Check sheet for the modelled part. Datum: model origin and axes. Units: mm. A direction names the side the tool comes from. Coordinates: 2 decimals unless noted, no trailing zeros. Write each loop counter-clockwise with the first axis right and the second up, starting at its lowest first coordinate (ties: lowest second). Pieces come first, ordered by that corner, then holes. Notation, with made-up numbers: (69, -3.5) - (97, -3.5) arc R14 ccw to (97, 11.5) - close; hole circle Ø9 at (43, 7). An arc over 180 degrees is marked (long way). Write each question's results on one line, items separated by ' | '.
from build123d import *

# Parameters (mm, degrees)
EXTRUDE_1_DEPTH          = 5
SKETCH_3_R               = 2
SKETCH_3_R_2             = 1
EXTRUDE_2_DEPTH          = 4
EXTRUDE_2_DEPTH_BACK     = 14
CUT_EXTRUDE_1_DEPTH      = 4
SKETCH_4_W               = 2.59101906
SKETCH_4_H               = 1.951015164
SKETCH_4_H_2             = 2.185859581
CUT_EXTRUDE_2_DEPTH      = 1
CUT_EXTRUDE_2_DEPTH_BACK = 22.850089698
SKETCH_5_W               = 31.280846128
SKETCH_5_H               = 26.509191634
CUT_EXTRUDE_3_DEPTH      = 10
CUT_EXTRUDE_4_DEPTH      = 10
EXTRUDE_4_DEPTH          = 10


with BuildPart() as part:
    # 草图1 → 凸台-拉伸1 (new body, symmetric)
    with BuildSketch(Plane.XY):
        with BuildLine():
            Line((-11, -0.656322646), (-11, -22.429975294))
            ThreePointArc((-11, -22.429975294), (-16.212842401, -27.826367541), (-21.786325372, -22.803314409))
            add(Edge.make_bspline(
                [(-20.992129713, -14.197793305), (-22.083985192, -18.508547069), (-21.786325372, -22.803314409)],
                knots=[0, 0, 0, 0.849528989, 0.849528989, 0.849528989], degree=2))
            add(Edge.make_bspline(
                [(-20.992129713, -14.197793305), (-19.982477614, -1.835246339), (-16.911295032, 22.315403308), (-5.101083491, 23.268557164)],
                knots=[0.325260196, 0.325260196, 0.325260196, 0.325260196, 1, 1, 1, 1], degree=3))
            Line((-5.101083491, 23.268557164), (-5.101083491, 16.3035208))
            ThreePointArc((-5.101083491, 16.3035208), (-5.344239377, 14.111719499), (-6.061882079, 12.026508076))
            Line((-6.061882079, 12.026508076), (-10.039201412, 3.620690077))
            ThreePointArc((-10.039201412, 3.620690077), (-10.756844114, 1.535478654), (-11, -0.656322646))
        make_face()
    extrude(amount=EXTRUDE_1_DEPTH, both=True)

    # 草图3 → 凸台-拉伸2 (add, two sides)
    with BuildSketch(Plane.XY.offset(5)) as extrude_2_sk:
        with Locations((-16.399623741, -22.429975294)):
            Circle(SKETCH_3_R)
        with Locations((-14.366531857, 0.706079338)):
            Circle(SKETCH_3_R_2)
    extrude(amount=EXTRUDE_2_DEPTH)
    extrude(extrude_2_sk.sketch, amount=-EXTRUDE_2_DEPTH_BACK)

    # 草图2 → 切除-拉伸1 (cut, symmetric)
    with BuildSketch(Plane.XY):
        with BuildLine():
            Line((-14.16063588, 12.808117781), (14.16063588, 12.808117781))
            add(Edge.make_bspline(
                [(14.16063588, 12.808117781), (18.7957473, 3.012389753), (18.151937314, -8.213759494), (19.7286529, -18.675237718)],
                knots=[0, 0, 0, 0, 1, 1, 1, 1], degree=3))
            Line((19.7286529, -18.675237718), (-19.7286529, -18.675237718))
            add(Edge.make_bspline(
                [(-14.16063588, 12.808117781), (-18.7957473, 3.012389753), (-18.151937314, -8.213759494), (-19.7286529, -18.675237718)],
                knots=[0, 0, 0, 0, 1, 1, 1, 1], degree=3))
        make_face()
    extrude(amount=CUT_EXTRUDE_1_DEPTH, both=True, mode=Mode.SUBTRACT)

    # 草图4 → 切除-拉伸2 (cut, two sides)
    with BuildSketch(Plane(origin=(0, 0, 0), x_dir=(0, 0, -1), z_dir=(1, 0, 0))) as cut_extrude_2_sk:
        with Locations((-6.29550953, -20.454467712)):
            Rectangle(SKETCH_4_W, SKETCH_4_H)
        with Locations((-6.29550953, -24.522905085)):
            Rectangle(SKETCH_4_W, SKETCH_4_H_2)
        with Locations((6.29550953, -24.522905085)):
            Rectangle(SKETCH_4_W, SKETCH_4_H_2)
        with Locations((6.29550953, -20.454467712)):
            Rectangle(SKETCH_4_W, SKETCH_4_H)
    extrude(amount=CUT_EXTRUDE_2_DEPTH, mode=Mode.SUBTRACT)
    extrude(cut_extrude_2_sk.sketch, amount=-CUT_EXTRUDE_2_DEPTH_BACK, mode=Mode.SUBTRACT)

    # 草图5 → 切除-拉伸3 (cut)
    with BuildSketch(Plane.XY.offset(5)):
        with Locations((-12.035980348, 17.707965105)):
            Rectangle(SKETCH_5_W, SKETCH_5_H)
    extrude(amount=-CUT_EXTRUDE_3_DEPTH, mode=Mode.SUBTRACT)

    # 草图6 → 切除-拉伸4 (cut)
    with BuildSketch(Plane.XY.offset(5)):
        with BuildLine():
            Line((-11, -1.030772695), (-7.289425252, 0))
            Line((-7.289425252, 0), (-6.627618858, 7.054774986))
            Line((-6.627618858, 7.054774986), (-15.000908449, 5.846258962))
            Line((-15.000908449, 5.846258962), (-16.238198664, 4.453369288))
            add(Edge.make_bspline(
                [(-16.238198664, 4.453369288), (-11.717955923, 3.797110984), (-11, -1.030772695)],
                knots=[0, 0, 0, 1, 1, 1], degree=2))
        make_face()
    extrude(amount=-CUT_EXTRUDE_4_DEPTH, mode=Mode.SUBTRACT)

    # 草图7 → 凸台-拉伸4 (add)
    with BuildSketch(Plane.XY.offset(5)):
        Polygon((-18.271249604, 4.453369288), (-18.271249604, 41.616361527), (-15.271249597, 41.616361527), (-15.271249604, 4.25345908), align=None)
    extrude(amount=-EXTRUDE_4_DEPTH)


solid = part.part
1. Access from +Z, -Z, +X, -X, +Y, -Y to the whole of each face (thin tool, end or side, straight path). Record for faces 5 (the cylindrical face through (-14.5, -21.8, -7.4)), 6 (the flat face through (-15.271, 23, 0)), 7 (the cylindrical face through (-14.5, -21.8, 7.4)), 8 (the flat face through (-11, -19, 0)), 9 (the flat face through (-16, -21.43, -6)).
Values follow:
face 5: -Z | face 6: +Z, -Z, +X, +Y | face 7: +Z | face 8: +Z, -Z, +X, +Y, -Y | face 9: +X, -X
2. Draft check along Z on faces 1 (the flat face through (-14, 1, -9)), 2 (the cylindrical face through (-15.366, 0.75, 6.972)), 3 (the flat face through (-14, 1, 9)), 4 (the flat face through (-15, -7, 4)). Enter one of: pulls with the +Z half, pulls with the -Z half, needs draft (parallel to the pull), parting line crosses it, or undercut.
Values follow:
face 1: pulls with the -Z half | face 2: needs draft | face 3: pulls with the +Z half | face 4: undercut
3. Sectioned sample at B-B (z = 6.25). Record the cut outline in (x, y), then the cut area to 3 significant figures.
Values follow:
outline: (-18.13, -23.43) - (-14.67, -23.43) arc R2 ccw to (-14.67, -21.43) - (-18.13, -21.43) arc R2 ccw to start; circle Ø2 at (-14.37, 0.71) | area: 10.8 mm^2
4. Material ranges on L1, parallel to Z at x = -12, y = -10; L2, parallel to Z at x = -16.25, y = 10; L3, parallel to Y at x = -16.25, z = -3, recorded low to high. Write a range as [from, to].
Values follow:
L1: z = [-5, -4], [4, 5] | L2: z = [-5, 5] | L3: y = [-27.83, -18.68], [4.32, 41.62]
5. Go/stop test with flat-tipped pins: pin 1 (4 mm diameter, centred on x = -15, z = 0.5, fed in from +Y); pin 2 (2.5 mm diameter, centred on x = -14.5, y = -9, fed in from -Z); pin 3 (3 mm diameter, centred on y = 32, z = -2, fed in from -X); pin 4 (5 mm diameter, centred on x = -19.5, z = -4, fed in from -Y). Record where each tip stops, or that it passes through.
Values follow:
pin 1: stops at y = 41.62 | pin 2: stops at z = -5 | pin 3: stops at x = -18.27 | pin 4: stops at y = -27.8
6. Sectioned sample at A-A (y = 21.5). Record the cut outline in (x, z).
Values follow:
outline: (-18.27, -5) - (-15.27, -5) - (-15.27, 5) - (-18.27, 5) - close
